Autodesk Inventor part; units mm, degrees
ref_plane "工作平面2" through (-3.5, 0, 4) normal (0, 1, 0) x (1, 0, 0)
ref_plane "YZ Plane" through (0, 0, 0) normal (1, 0, 0) x (0, 1, 0)
ref_plane "XZ Plane" through (0, 0, 0) normal (0, 1, 0) x (-1, 0, 0)
sketch "草圖1" plane through (0, 0, 0) normal (0, 0, 1) x (1, 0, 0)
  line L0 (-20, 6.5) -> (20, 6.5)
  line L1 (20, 6.5) -> (20, -6.5)
  line L2 (20, -6.5) -> (-20, -6.5)
  line L3 (-20, -6.5) -> (-20, 6.5)
  line L4 (-20, 6.5) -> (20, -6.5) construction
  line L5 (20, 6.5) -> (-20, -6.5) construction
  circle A0 centre (-9.4, 0) radius 2.8
  circle A1 centre (9.4, 0) radius 2.8
  point P0 (0, 0)
  dimension "d0" = 40
  dimension "d1" = 13
  dimension "d2" = 5.6
  dimension "d3" = 5.6
extrude "擠出1" add sketch "草圖1" along normal blind 4
sketch "草圖3" plane through (0, 0, 4) normal (0, 0, 1) x (1, 0, 0)
  line L0 (3.5, -3.5) -> (-3.5, -3.5)
  line L1 (-3.5, -3.5) -> (-3.5, 3.5)
  line L2 (-3.5, 3.5) -> (3.5, 3.5)
  line L3 (3.5, 3.5) -> (3.5, -3.5)
  line L4 (3.5, -3.5) -> (-3.5, 3.5) construction
  line L5 (-3.5, -3.5) -> (3.5, 3.5) construction
  point P0 (0, 0)
  dimension "d8" = 7
  dimension "d9" = 7
extrude "擠出2" add sketch "草圖3" along normal blind 33
ref_plane "工作平面2" through (-3.5, 0, 4) normal (0, 1, 0) x (1, 0, 0)
sketch "草圖4" plane through (-3.5, 0, 4) normal (0, 1, 0) x (1, 0, 0)
  circle A0 centre (4.1663, -39.5) radius 9.5
  circle A1 centre (4.1663, -39.5) radius 6.5
  dimension "d14" = 19
  dimension "d15" = 13
extrude "擠出3" add sketch "草圖4" along normal mid plane 7
properties part number "T字形固定件"
Source: CAD feature listing. Evaluate the final solid. Frame: model axes, mm. A direction names the side the tool comes from. Round coordinates to 2 decimals unless told otherwise and drop trailing zeros. Loops run counter-clockwise (first coordinate to the right, second up) from the corner with the lowest first, then second, coordinate; pieces in that order, holes last. Notation, with made-up numbers: M -19.5,-27.5 L 30.5,-27.5 A28 ccw 30.5,0.5 Z; hole C -33.5,77.5 d1. An arc over 180 degrees is marked long. Put each result on its own line as item: value.
(1) Section A-A, the plane y = 0. Return loops of the section in (x, z).
Solutions:
outline: M -20,0 L -12.2,0 L -12.2,4 L -20,4 Z; M -6.6,0 L 6.6,0 L 6.6,4 L 3.5,4 L 3.5,34.43 A9.5 ccw long -3.5,34.96 L -3.5,4 L -6.6,4 Z; M 12.2,0 L 20,0 L 20,4 L 12.2,4 Z; hole C 0.67,43.5 d13
(2) Access query for faces 4 (the face through (1, -3.5, 28)), 5 (the face through (1, 3.5, 28)), 6 (the face through (-12.2, -0.1, 2)), 7 (the face through (-3.5, 0, 19)). Directions: +Z, -Z, +X, -X, +Y, -Y. A direction counts if a zero-diameter tool reaches every point of the face in a straight line with its end or side. Return the directions, or none.
Solutions:
face 4: +Z, +X, -X, -Y
face 5: +Z, +X, -X, +Y
face 6: -Z
face 7: -X, +Y, -Y
(3) Section C-C, the plane z = 43.5. Return loops of the section in (x, y), and give its area (3 significant figures).
Solutions:
outline: M -8.83,-3.5 L -5.83,-3.5 L -5.83,3.5 L -8.83,3.5 Z; M 7.17,-3.5 L 10.17,-3.5 L 10.17,3.5 L 7.17,3.5 Z
area: 42.0 mm²
(4) First-contact query: pin 1 (12 mm diameter, centred on x = 9.5, z = 44.5, fed in from +Y); pin 2 (4 mm diameter, centred on y = 5, z = 35, fed in from -X); pin 3 (5 mm diameter, centred on y = 0.5, z = 25.5, fed in from +X). Flat tips, straight axial feed; report the tip coordinate or a pass-through.
Solutions:
pin 1: y = 3.5
pin 2: x = -5.56
pin 3: x = 3.5
(5) Pull-direction query (X, two-part tool) for faces 1 (the face through (3.5, 0, 19)), 2 (the face through (-0.743, -0.049, 37.155)), 3 (the face through (0, -4, 4)); classes: released by +X, released by -X, zero draft, split by the parting line, or undercut.
Solutions:
face 1: released by +X
face 2: undercut
face 3: zero draft
(6) Section D-D, the plane x = 9.4. Return loops of the section in (y, z), and give its area (3 significant figures).
Solutions:
outline: M -6.5,0 L -2.8,0 L -2.8,4 L -6.5,4 Z; M -3.5,39.76 L 3.5,39.76 L 3.5,47.24 L -3.5,47.24 Z; M 2.8,0 L 6.5,0 L 6.5,4 L 2.8,4 Z
area: 81.9 mm²
(7) Section B-B, the plane x = -9.4. Return loops of the section in (y, z).
Solutions:
outline: M -6.5,0 L -2.8,0 L -2.8,4 L -6.5,4 Z; M 2.8,0 L 6.5,0 L 6.5,4 L 2.8,4 Z
(8) Ray query, line 1 (Y direction, x = -9.4, z = 2.8); line 2 (X direction, y = -1.25, z = 43.5); line 3 (Z direction, x = 2, y = -5.25). Return the intervals inside material, ascending. Write a range as [from, to].
Solutions:
line 1: [-6.5, -2.8], [2.8, 6.5]
line 2: [-8.83, -5.83], [7.17, 10.17]
line 3: [0, 4]
